Here's how the part is built. I have some questions about the finished solid (model axes, mm). A direction names the side the tool comes from. Coordinates: 2 decimals unless noted, no trailing zeros. Order: outer loops, then holes, each group sorted by start corner. A loop starts at its lowest first (then second) coordinate and runs counter-clockwise, first axis right, second up. Notation, with made-up numbers: (22.25, 30) - (75.25, 30) arc R14 cw to (75.25, 35) - close; hole circle Ø3 at (67.25, 9). An arc over 180 degrees is marked (long way). Answer in a Markdown table with one row per item. Add a question column.
Item 1: On a 3-axis mill with a long thin cutter (end or side, diameter ignored), from which of +Z, -Z, +X, -X, +Y, -Y can I reach the whole of each face in a straight line? I mean faces 1 (the flat face through (-10, 20, -349.25)), 2 (the cylindrical face through (-6.508, 16.092, -172.18)), 3 (the flat face through (0, 3, -172)). Say none if no direction works.
Item 2: Thinking about a two-plate mould opening in Y: for faces 4 (the flat face through (-15, 34.925, -172)), 5 (the flat face through (1.27, 3, -172)), 6 (the flat face through (-15, 33.655, -172)), which applies, +Y half, -Y half, draft (parallel to the pull), parting line (faces both ways), or undercut?
Item 3: Will these pins go through, and if not, where does the flat tip stop? pin 1 Ø2 at (y, z) = (20.5, -207.5) entering from +X; pin 2 Ø5 at (y, z) = (13.5, -104.5) entering from +X; pin 3 Ø6 at (y, z) = (8, -297) entering from -X.
Item 4: I want a section at B-B (y = 16.5). Please give me the cut outline in (x, z), plus the area to 3 significant figures.
Item 5: If I drill on line 1 along Y through (x, z) = (-20, -312) (3 decimals); line 2 along Y through (x, z) = (-2.25, -323.5); line 3 along X through (y, z) = (2.5, -157.5), over which ranges is the centre line in solid material (lowest first)? Write a range as from..to.
```python
from build123d import *

# Parameters (mm, degrees)
EXTRUDE_THIN1_DEPTH = 349.25
FILLET1_R           = 1.27


with BuildPart() as part:
    # Sketch1 → Extrude-Thin1 (new body)
    with BuildSketch(Plane.XY):
        with BuildLine():
            Line((0, 0), (0, 5.55625))
            Line((0, 5.55625), (-6.35, 5.55625))
            Line((-6.35, 5.55625), (-6.35, 10.31875))
            ThreePointArc((-6.35, 10.31875), (-7.597327769, 15.43402449), (-11.059297297, 19.400966216))
            Line((-11.059297297, 19.400966216), (-13.654216216, 21.230452703))
            ThreePointArc((-13.654216216, 21.230452703), (-16.453819125, 24.438413231), (-17.4625, 28.575))
            Line((-17.4625, 28.575), (-22.225, 28.575))
            Line((-22.225, 28.575), (-22.225, 34.925))
            Line((-22.225, 34.925), (-8.73125, 34.925))
            Line((-8.73125, 34.925), (-8.73125, 33.655))
            Line((-8.73125, 33.655), (-20.955, 33.655))
            Line((-20.955, 33.655), (-20.955, 29.845))
            Line((-20.955, 29.845), (-16.087271104, 29.845))
            ThreePointArc((-16.087271104, 29.845), (-15.596279625, 25.600802309), (-12.922421622, 22.26842027))
            Line((-12.922421622, 22.26842027), (-10.327502703, 20.438933784))
            ThreePointArc((-10.327502703, 20.438933784), (-6.469879514, 16.018627289), (-5.08, 10.31875))
            Line((-5.08, 10.31875), (-5.08, 6.82625))
            Line((-5.08, 6.82625), (1.27, 6.82625))
            Line((1.27, 6.82625), (1.27, 0))
            Line((1.27, 0), (0, 0))
        make_face()
    extrude(amount=-EXTRUDE_THIN1_DEPTH)

    # Fillet1
    fillet1_edges = [part.edges().sort_by_distance(p)[0] for p in [
        (-16.087271104, 29.845, -174.625),
        (1.27, 6.82625, -174.625),
        (-6.35, 5.55625, -174.625),
        (-22.225, 28.575, -174.625),
        (-22.225, 34.925, -174.625),
    ]]
    fillet(fillet1_edges, radius=FILLET1_R)


solid = part.part
```
Values follow:
| question | item | result |
|---|---|---|
| 1 | face 1 | -Z, +X, -X, +Y, -Y |
| 1 | face 2 | +Z, -Z, +X |
| 1 | face 3 | +Z, -Z, -X, -Y |
| 2 | face 4 | +Y half |
| 2 | face 5 | draft |
| 2 | face 6 | undercut |
| 3 | pin 1 | stops at x = -9.15 |
| 3 | pin 2 | stops at x = -5.1 |
| 3 | pin 3 | stops at x = -6.37 |
| 4 | outline | (-8.23, -349.25) - (-6.73, -349.25) - (-6.73, 0) - (-8.23, 0) - close |
| 4 | area | 522 mm^2 |
| 5 | line 1 | y = 28.575..29.845, 33.655..34.925 |
| 5 | line 2 | y = 5.56..6.83 |
| 5 | line 3 | x = 0..1.27 |
